The listing builds one solid part. Answer for the finished solid, in the listing's coordinates (mm). Round coordinates to 2 decimals unless told otherwise and drop trailing zeros.
Item 1: Each of these flat-tipped pins is pushed along its axis until it touches: pin 1 (5 mm diameter, centred on y = -20, z = -1895, fed in from +X); pin 2 (8.5 mm diameter, centred on x = -1.5, z = -1407, fed in from -Y); pin 3 (4 mm diameter, centred on x = 2, y = 31.5, fed in from +Z); pin 4 (2.5 mm diameter, centred on y = 38.5, z = -1913.5, fed in from -X). Where does it stop, or does it pass through?
Item 2: Find section A-A on z = -498.5. Give the number of separate pieces and of enclosed holes in the cut face, then the cut area to 3 significant figures.
Item 3: Find the intervals of material crossed by probe 1 along X at (y, z) = (26.5, -552.5); probe 2 along Y at (x, z) = (-9.5, -458.5); probe 3 along Y at (x, z) = (0, -2461.5), in increasing order.
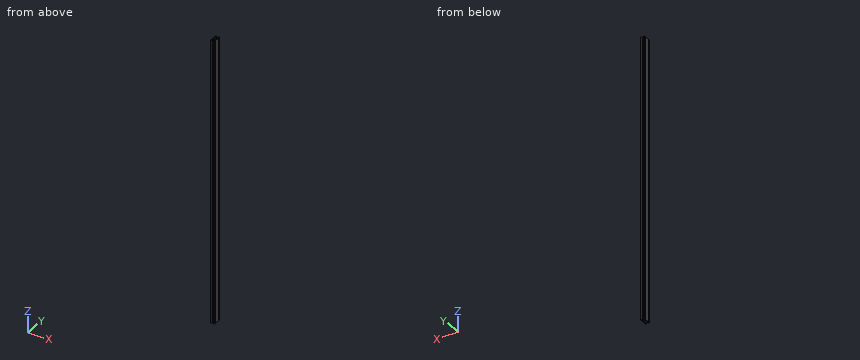
```python
from build123d import *

# Parameters (mm, degrees)
SKETCH1_R           = 2.5
SKETCH1_R_2         = 6
BOSS_EXTRUDE1_DEPTH = 2900


with BuildPart() as part:
    # Sketch1 → Boss-Extrude1 (new body)
    with BuildSketch(Plane.XY):
        with BuildLine():
            Line((-17, -40), (-4.1, -40))
            Line((-4.1, -40), (-4.1, -37))
            Line((-4.1, -37), (-10.5, -37))
            Line((-10.5, -37), (-10.5, -33.6627417))
            ThreePointArc((-10.5, -33.6627417), (-10.378207252, -33.050448208), (-10.03137085, -32.53137085))
            Line((-10.03137085, -32.53137085), (-7.464466094, -29.964466094))
            ThreePointArc((-7.464466094, -29.964466094), (-5.84234935, -28.880602337), (-3.928932188, -28.5))
            Line((-3.928932188, -28.5), (3.928932188, -28.5))
            ThreePointArc((3.928932188, -28.5), (5.84234935, -28.880602337), (7.464466094, -29.964466094))
            Line((7.464466094, -29.964466094), (10.03137085, -32.53137085))
            ThreePointArc((10.03137085, -32.53137085), (10.378207252, -33.050448208), (10.5, -33.6627417))
            Line((10.5, -33.6627417), (10.5, -37))
            Line((10.5, -37), (4.1, -37))
            Line((4.1, -37), (4.1, -40))
            Line((4.1, -40), (17, -40))
            ThreePointArc((17, -40), (19.121320344, -39.121320344), (20, -37))
            Line((20, -37), (20, -24.1))
            Line((20, -24.1), (17, -24.1))
            Line((17, -24.1), (17, -30.5))
            Line((17, -30.5), (13.6627417, -30.5))
            ThreePointArc((13.6627417, -30.5), (13.050448208, -30.378207252), (12.53137085, -30.03137085))
            Line((12.53137085, -30.03137085), (9.964466094, -27.464466094))
            ThreePointArc((9.964466094, -27.464466094), (8.880602337, -25.84234935), (8.5, -23.928932188))
            Line((8.5, -23.928932188), (8.5, -16.071067812))
            ThreePointArc((8.5, -16.071067812), (8.880602337, -14.15765065), (9.964466094, -12.535533906))
            Line((9.964466094, -12.535533906), (12.53137085, -9.96862915))
            ThreePointArc((12.53137085, -9.96862915), (13.050448208, -9.621792748), (13.6627417, -9.5))
            Line((13.6627417, -9.5), (17, -9.5))
            Line((17, -9.5), (17, -15.9))
            Line((17, -15.9), (20, -15.9))
            Line((20, -15.9), (20, 15.9))
            Line((20, 15.9), (17, 15.9))
            Line((17, 15.9), (17, 9.5))
            Line((17, 9.5), (13.6627417, 9.5))
            ThreePointArc((13.6627417, 9.5), (13.050448208, 9.621792748), (12.53137085, 9.96862915))
            Line((12.53137085, 9.96862915), (9.964466094, 12.535533906))
            ThreePointArc((9.964466094, 12.535533906), (8.880602337, 14.15765065), (8.5, 16.071067812))
            Line((8.5, 16.071067812), (8.5, 23.928932188))
            ThreePointArc((8.5, 23.928932188), (8.880602337, 25.84234935), (9.964466094, 27.464466094))
            Line((9.964466094, 27.464466094), (12.53137085, 30.03137085))
            ThreePointArc((12.53137085, 30.03137085), (13.050448208, 30.378207252), (13.6627417, 30.5))
            Line((13.6627417, 30.5), (17, 30.5))
            Line((17, 30.5), (17, 24.1))
            Line((17, 24.1), (20, 24.1))
            Line((20, 24.1), (20, 37))
            ThreePointArc((20, 37), (19.121320344, 39.121320344), (17, 40))
            Line((17, 40), (4.1, 40))
            Line((4.1, 40), (4.1, 37))
            Line((4.1, 37), (10.5, 37))
            Line((10.5, 37), (10.5, 33.6627417))
            ThreePointArc((10.5, 33.6627417), (10.378207252, 33.050448208), (10.03137085, 32.53137085))
            Line((10.03137085, 32.53137085), (7.464466094, 29.964466094))
            ThreePointArc((7.464466094, 29.964466094), (5.84234935, 28.880602337), (3.928932188, 28.5))
            Line((3.928932188, 28.5), (-3.928932188, 28.5))
            ThreePointArc((-3.928932188, 28.5), (-5.84234935, 28.880602337), (-7.464466094, 29.964466094))
            Line((-7.464466094, 29.964466094), (-10.03137085, 32.53137085))
            ThreePointArc((-10.03137085, 32.53137085), (-10.378207252, 33.050448208), (-10.5, 33.6627417))
            Line((-10.5, 33.6627417), (-10.5, 37))
            Line((-10.5, 37), (-4.1, 37))
            Line((-4.1, 37), (-4.1, 40))
            Line((-4.1, 40), (-17, 40))
            ThreePointArc((-17, 40), (-19.121320344, 39.121320344), (-20, 37))
            Line((-20, 37), (-20, 24.1))
            Line((-20, 24.1), (-17, 24.1))
            Line((-17, 24.1), (-17, 30.5))
            Line((-17, 30.5), (-13.6627417, 30.5))
            ThreePointArc((-13.6627417, 30.5), (-13.050448208, 30.378207252), (-12.53137085, 30.03137085))
            Line((-12.53137085, 30.03137085), (-9.964466094, 27.464466094))
            ThreePointArc((-9.964466094, 27.464466094), (-8.880602337, 25.84234935), (-8.5, 23.928932188))
            Line((-8.5, 23.928932188), (-8.5, 16.071067812))
            ThreePointArc((-8.5, 16.071067812), (-8.880602337, 14.15765065), (-9.964466094, 12.535533906))
            Line((-9.964466094, 12.535533906), (-12.53137085, 9.96862915))
            ThreePointArc((-12.53137085, 9.96862915), (-13.050448208, 9.621792748), (-13.6627417, 9.5))
            Line((-13.6627417, 9.5), (-17, 9.5))
            Line((-17, 9.5), (-17, 15.9))
            Line((-17, 15.9), (-20, 15.9))
            Line((-20, 15.9), (-20, -15.9))
            Line((-20, -15.9), (-17, -15.9))
            Line((-17, -15.9), (-17, -9.5))
            Line((-17, -9.5), (-13.6627417, -9.5))
            ThreePointArc((-13.6627417, -9.5), (-13.050448208, -9.621792748), (-12.53137085, -9.96862915))
            Line((-12.53137085, -9.96862915), (-9.964466094, -12.535533906))
            ThreePointArc((-9.964466094, -12.535533906), (-8.880602337, -14.15765065), (-8.5, -16.071067812))
            Line((-8.5, -16.071067812), (-8.5, -23.928932188))
            ThreePointArc((-8.5, -23.928932188), (-8.880602337, -25.84234935), (-9.964466094, -27.464466094))
            Line((-9.964466094, -27.464466094), (-12.53137085, -30.03137085))
            ThreePointArc((-12.53137085, -30.03137085), (-13.050448208, -30.378207252), (-13.6627417, -30.5))
            Line((-13.6627417, -30.5), (-17, -30.5))
            Line((-17, -30.5), (-17, -24.1))
            Line((-17, -24.1), (-20, -24.1))
            Line((-20, -24.1), (-20, -37))
            ThreePointArc((-20, -37), (-19.121320344, -39.121320344), (-17, -40))
        make_face()
        with Locations((15, 35)):
            Circle(SKETCH1_R, mode=Mode.SUBTRACT)
        with Locations((15, -35)):
            Circle(SKETCH1_R, mode=Mode.SUBTRACT)
        with Locations((0, 20)):
            Circle(SKETCH1_R_2, mode=Mode.SUBTRACT)
        with Locations((0, -20)):
            Circle(SKETCH1_R_2, mode=Mode.SUBTRACT)
        with Locations((-15, 35)):
            Circle(SKETCH1_R, mode=Mode.SUBTRACT)
        with Locations((-15, -35)):
            Circle(SKETCH1_R, mode=Mode.SUBTRACT)
        with BuildLine():
            Line((-14.242640687, -4.242640687), (-9.949747468, -8.535533906))
            ThreePointArc((-9.949747468, -8.535533906), (-8.327630724, -9.619397663), (-6.414213562, -10))
            Line((-6.414213562, -10), (6.414213562, -10))
            ThreePointArc((6.414213562, -10), (8.327630724, -9.619397663), (9.949747468, -8.535533906))
            Line((9.949747468, -8.535533906), (14.242640687, -4.242640687))
            ThreePointArc((14.242640687, -4.242640687), (16, 0), (14.242640687, 4.242640687))
            Line((14.242640687, 4.242640687), (9.949747468, 8.535533906))
            ThreePointArc((9.949747468, 8.535533906), (8.327630724, 9.619397663), (6.414213562, 10))
            Line((6.414213562, 10), (-6.414213562, 10))
            ThreePointArc((-6.414213562, 10), (-8.327630724, 9.619397663), (-9.949747468, 8.535533906))
            Line((-9.949747468, 8.535533906), (-14.242640687, 4.242640687))
            ThreePointArc((-14.242640687, 4.242640687), (-16, 0), (-14.242640687, -4.242640687))
        make_face(mode=Mode.SUBTRACT)
    extrude(amount=-BOSS_EXTRUDE1_DEPTH)


solid = part.part
```
Check values:
1. pin 1: stops at x = 8.5
1. pin 2: stops at y = -40
1. pin 3: passes through
1. pin 4: stops at x = -19.99
2. separate pieces: 1
2. enclosed holes: 7
2. area: 1,280 mm2
3. probe 1: x = -20 to -17, -9.21 to 9.21, 17 to 20
3. probe 2: y = -40 to -37, -32 to -26.93, -13.07 to -8.93, 8.93 to 13.07, 26.93 to 32, 37 to 40
3. probe 3: y = -28.5 to -26, -14 to -10, 10 to 14, 26 to 28.5
